Could you check a few things on this model? Use its own coordinates, in mm. Give positions to 0.01 mm unless a question says otherwise; leave off trailing zeros. Loops run counter-clockwise (first coordinate to the right, second up) from the corner with the lowest first, then second, coordinate; pieces in that order, holes last. Notation, with made-up numbers: M 16.5,-17.75 L 20.5,-17.75 A27 ccw 20.5,14.25 Z; hole C 10.25,46 d1. An arc over 180 degrees is marked long. Answer in a Markdown table with one row per item. Add a question column.
1. I need wall thicknesses on line 1 along X through (y, z) = (-6, 1.35); line 2 along X through (y, z) = (-8, 3.5); line 3 along Y through (x, z) = (283, 3.6). Which ranges of each line are inside material? Lowest first, please. Write a range as from..to.
2. If we section it at A-A on y = 0: List the corners of the cut face in (x, z) for me (3 decimals).
3. If we section it at B-B on z = 0.95: List the corners of the cut face in (x, y) for me (3 decimals), then the cut area to 3 significant figures.
4. I'm going to push flat-ended pins straight in: pin 1 Ø2 at (x, z) = (200, 2) entering from -Y; pin 2 Ø1.5 at (y, z) = (9.5, 2) entering from -X; pin 3 Ø11.5 at (x, y) = (330, 0) entering from -Z; pin 4 Ø2 at (x, z) = (36.5, 1.5) entering from -Y. Where does each tip first touch, or does it pass through?
5. If we section it at D-D on x = 330: List the corners of the cut face in (y, z) for me (3 decimals).
6. If we section it at C-C on y = -14: List the corners of the cut face in (x, z) for me.
```python
from build123d import *

# Parameters (mm, degrees)
SKETCH_1_R      = 9.525
EXTRUDE_1_DEPTH = 4
FILLET_1_R      = 20


with BuildPart() as part:
    # 草图1 → 凸台-拉伸1 (new body)
    with BuildSketch(Plane.XY):
        with BuildLine():
            Line((-4.63962822, 36.550100793), (334.63962822, 36.550100793))
            Line((334.63962822, 36.550100793), (347.382944688, 7.670282522))
            ThreePointArc((347.382944688, 7.670282522), (337.670282522, -17.382944688), (312.617055312, -7.670282522))
            Line((312.617055312, -7.670282522), (301.929730112, 16.550100793))
            Line((301.929730112, 16.550100793), (28.070269888, 16.550100793))
            Line((28.070269888, 16.550100793), (17.382944688, -7.670282522))
            ThreePointArc((17.382944688, -7.670282522), (-7.670282522, -17.382944688), (-17.382944688, 7.670282522))
            Line((-17.382944688, 7.670282522), (-4.63962822, 36.550100793))
        make_face()
        Circle(SKETCH_1_R, mode=Mode.SUBTRACT)
        with Locations((330, 0)):
            Circle(SKETCH_1_R, mode=Mode.SUBTRACT)
    extrude(amount=EXTRUDE_1_DEPTH)

    # 圆角1
    fillet_1_edges = [part.edges().sort_by_distance(p)[0] for p in [
        (-4.63962822, 36.550100793, 2),
        (334.63962822, 36.550100793, 2),
        (301.929730112, 16.550100793, 2),
        (28.070269888, 16.550100793, 2),
    ]]
    fillet(fillet_1_edges, radius=FILLET_1_R)


solid = part.part
```
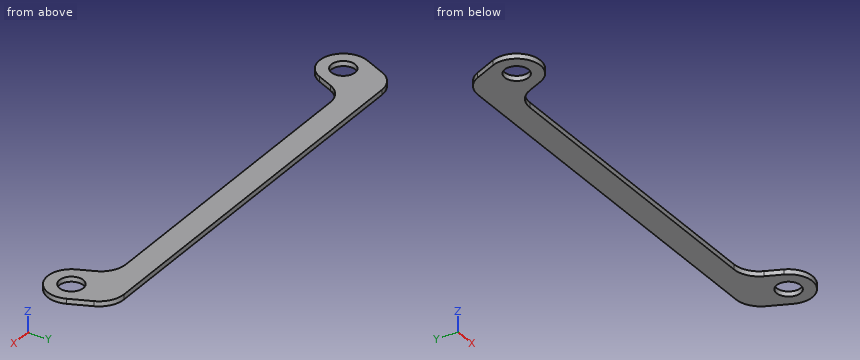
Results:
| question | item | result |
|---|---|---|
| 1 | line 1 | -18.03..-7.4, 7.4..18.12, 311.88..322.6, 337.4..348.03 |
| 1 | line 2 | -17.23..-5.17, 5.17..17.23, 312.77..324.83, 335.17..347.23 |
| 1 | line 3 | 16.55..36.55 |
| 2 | outline | M -19,0 L -9.525,0 L -9.525,4 L -19,4 Z; M 9.525,0 L 20.767,0 L 20.767,4 L 9.525,4 Z; M 309.233,0 L 320.475,0 L 320.475,4 L 309.233,4 Z; M 339.525,0 L 349,0 L 349,4 L 339.525,4 Z |
| 3 | outline | M -17.383,7.67 A19 ccw 17.383,-7.67 L 22.808,4.624 A20 cw 41.106,16.55 L 288.894,16.55 A20 cw 307.192,4.624 L 312.617,-7.67 A19 ccw 347.383,7.67 L 339.902,24.624 A20 ccw 321.604,36.55 L 8.396,36.55 A20 ccw -9.902,24.624 Z; hole C 0,0 d19.05; hole C 330,0 d19.05 |
| 3 | area | 8,900 mm2 |
| 4 | pin 1 | y = 16.55 |
| 4 | pin 2 | x = -16.91 |
| 4 | pin 3 | through |
| 4 | pin 4 | y = 15.75 |
| 5 | outline | M -19,0 L -9.525,0 L -9.525,4 L -19,4 Z; M 9.525,0 L 34.703,0 L 34.703,4 L 9.525,4 Z |
| 6 | outline | M -12.85,0 L 12.85,0 L 12.85,4 L -12.85,4 Z; M 317.15,0 L 342.85,0 L 342.85,4 L 317.15,4 Z |
